Work out the finished part from the listing and answer in its coordinate system (mm). Face numbers are marked on the shaded views. Give positions to 0.01 mm unless a question says otherwise; leave off trailing zeros. Write each loop counter-clockwise with the first axis right and the second up, starting at its lowest first coordinate (ties: lowest second). Pieces come first, ordered by that corner, then holes.
1) Straight lines are drawn through the part: probe 1 along X at (y, z) = (-2, 0.5); probe 2 along Y at (x, z) = (8.5, 2.5); probe 3 along X at (y, z) = (0, -0.25). For each, find the intervals that lie inside material, in ascending order.
2) Find section B-B (z = 0). Determine the outline of the cut face in (x, y), plus the area to 3 significant figures.
3) Determine the mould class of the marked faces 1, 2 and 3 for opening direction Z: pulls with the +Z half, pulls with the -Z half, needs draft (parallel to the pull), parting line crosses it, or undercut.
4) Given pin 1 Ø5 at (x, z) = (2, -3.5) entering from -Y; pin 2 Ø4 at (x, z) = (7.5, -2) entering from -Y; pin 3 Ø4 at (x, y) = (10, -3) entering from -Z; pin 4 Ø4 at (x, z) = (6, 0.5) entering from -Y, each flat-ended and moving along its own axis, determine where each tip first touches the part or whether it passes through.
5) Find section D-D (z = -3.5). Determine the outline of the cut face in (x, y), plus the area to 3 significant figures.
6) Find section A-A (x = 8.5). Determine the outline of the cut face in (y, z).
Autodesk Inventor part; units mm, degrees
ref_plane "YZ Plane" through (0, 0, 0) normal (1, 0, 0) x (0, 1, 0)
ref_plane "XZ Plane" through (0, 0, 0) normal (0, 1, 0) x (-1, 0, 0)
ref_plane "XY Plane" through (0, 0, 0) normal (0, 0, 1) x (1, 0, 0)
sketch "Sketch1" plane through (0, 0, 0) normal (0, 0, 1) x (1, 0, 0)
  line L0 (0, 0) -> (12.07, 0)
  line L1 (12.07, 0) -> (12.07, 5)
  line L2 (12.07, 5) -> (8.07, 5)
  line L3 (8.07, 5) -> (8.07, 3.9)
  line L4 (8.07, 3.9) -> (0, 3.9)
  line L5 (0, 3.9) -> (0, 0)
  dimension "d0" = 7.8
  dimension "d1" = 8.07
  dimension "d2" = 4
  dimension "d3" = 10
revolve "Revolution1" add sketch "Sketch1" angle 360 about axis through (0, 0, 0) along (1, 0, 0)
thread "Thread1"
sketch "Sketch2" plane through (12.07, 0, 0) normal (1, 0, 0) x (0, 0, -1)
  circle A0 centre (0, 0) radius 2.75
  circle A1 centre (0, 0) radius 1.05
  dimension "d7" = 5.5
  dimension "d8" = 2.1
extrude "Extrusion1" cut sketch "Sketch2" against normal blind 4
fillet "Fillet1" radius 1.05 1 edges at (12.07, 0, 1.05)
properties part number "DC Jack"
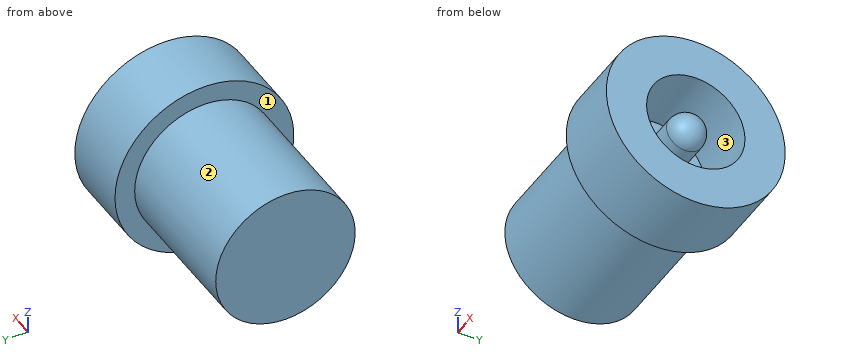
Results:
1. probe 1: x = 0 to 8.07
1. probe 2: y = -4.33 to -1.15, 1.15 to 4.33
1. probe 3: x = 0 to 12.04
2. outline: (0, -3.9) - (8.07, -3.9) - (8.07, -5) - (12.07, -5) - (12.07, -2.75) - (8.07, -2.75) - (8.07, -1.05) - (11.02, -1.05) arc R1.05 ccw to (11.02, 1.05) - (8.07, 1.05) - (8.07, 2.75) - (12.07, 2.75) - (12.07, 5) - (8.07, 5) - (8.07, 3.9) - (0, 3.9) - close
2. area: 88.9 mm2
3. face 1: needs draft
3. face 2: parting line crosses it
3. face 3: undercut
4. pin 1: stops at y = -3.77
4. pin 2: stops at y = -5
4. pin 3: stops at z = -4.9
4. pin 4: stops at y = -3.9
5. outline: (0, -1.72) - (8.07, -1.72) - (8.07, -3.57) - (12.07, -3.57) - (12.07, 3.57) - (8.07, 3.57) - (8.07, 1.72) - (0, 1.72) - close
5. area: 56.3 mm2
6. outline: circle Ø10 at (0, 0); circle Ø2.1 at (0, 0); hole circle Ø5.5 at (0, 0)
